Part model, mm, in its own coordinate system. Face numbers are marked on the shaded views. Coordinates: 2 decimals unless noted, no trailing zeros. Loops run counter-clockwise (first coordinate to the right, second up) from the corner with the lowest first, then second, coordinate; pieces in that order, holes last. Notation, with made-up numbers: M 38.25,-20 L 93.25,-20 A18 cw 93.25,10 Z; hole C 51.25,72.25 d7. An arc over 180 degrees is marked long. Use a Markdown table: item, result. Add a question column.
1) Pull direction Z, two halves, no side cores. Call the marked faces 1, 2 and 3: released by +Z, released by -Z, zero draft, split by the parting line, or undercut.
2) Wall check: probe 1 along Z at (x, y) = (-23, 44.5); probe 2 along X at (y, z) = (24, -3.5); probe 3 along Z at (x, y) = (2.5, 45). Give the ranges that are in metal, low to high. Write a range as from..to.
3) Band-saw the part on D-D (y = 47.5). List the corners of the cut face in (x, z), plus the area to 3 significant figures.
4) Band-saw the part on B-B (y = 29). List the corners of the cut face in (x, z).
5) Band-saw the part on A-A (z = -2.5). List the corners of the cut face in (x, y).
6) Pin check, flat tips, straight feed: pin 1 Ø2 at (x, z) = (3.5, -2) entering from -Y; pin 2 Ø1.5 at (x, z) = (16.5, -1.5) entering from -Y. Stop position of each tip, or through.
7) Band-saw the part on C-C (z = 1). List the corners of the cut face in (x, y), plus the area to 3 significant figures.
from build123d import *

# Parameters (mm, degrees)
F0_W     = 50
F0_H     = 25
F1_DEPTH = 50
F2_R     = 5
F3_R     = 5
F4_DEPTH = 50.001


with BuildPart() as f1:
    # F0 (on Front) → F1 (new body)
    with BuildSketch(Plane.XZ):
        Rectangle(F0_W, F0_H)
    extrude(amount=-F1_DEPTH)

    # F2
    f2_edges = [f1.edges().sort_by_distance(p)[0] for p in [
        (-25, 25, 12.5),
        (25, 25, 12.5),
        (0, 0, 12.5),
        (0, 50, 12.5),
    ]]
    fillet(f2_edges, radius=F2_R)

    # F3 (on face) → F4 (cut, through all)
    with BuildSketch(Plane(origin=(0, 50, 0), x_dir=(-1, 0, 0), z_dir=(0, 1, 0))):
        with Locations((-6.507594, -2.5)):
            Circle(F3_R)
    extrude(amount=-F4_DEPTH, mode=Mode.SUBTRACT)


solid = f1.part
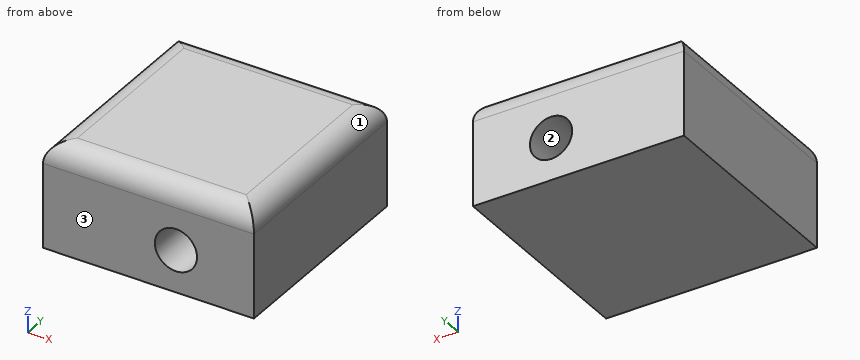
Entries:
| question | item | result |
|---|---|---|
| 1 | face 1 | released by +Z |
| 1 | face 2 | undercut |
| 1 | face 3 | zero draft |
| 2 | probe 1 | -12.5..11.5 |
| 2 | probe 2 | -25..1.61, 11.41..25 |
| 2 | probe 3 | -12.5..-5.49, 0.49..12.5 |
| 3 | outline | M -25,-12.5 L 25,-12.5 L 25,7.5 A5 ccw 22.5,11.83 L -22.5,11.83 A5 ccw -25,7.5 Z; hole C 6.51,-2.5 d10 |
| 3 | area | 1,130 mm2 |
| 4 | outline | M -25,-12.5 L 25,-12.5 L 25,7.5 A5 ccw 20,12.5 L -20,12.5 A5 ccw -25,7.5 Z; hole C 6.51,-2.5 d10 |
| 5 | outline | M -25,0 L 1.51,0 L 1.51,50 L -25,50 Z; M 11.51,0 L 25,0 L 25,50 L 11.51,50 Z |
| 6 | pin 1 | through |
| 6 | pin 2 | y = 0 |
| 7 | outline | M -25,0 L 2.94,0 L 2.94,50 L -25,50 Z; M 10.08,0 L 25,0 L 25,50 L 10.08,50 Z |
| 7 | area | 2,140 mm2 |
